The figure shows three views and two pictorial views of one solid part (mm, origin at its lowest corner). Answer the questions. A direction names the side the tool comes from. Coordinates: 2 decimals unless noted, no trailing zeros. Order: outer loops, then holes, each group sorted by start corner. A loop starts at its lowest first (then second) coordinate and runs counter-clockwise, first axis right, second up. Notation, with made-up numbers: (4, 30.25) -> (60, 30.25) arc R23 cw to (60, 44.25) -> close; hole circle Ø9 at (64, -28). An arc over 180 degrees is marked (long way). Return JSON: item names as keys, results as strings.
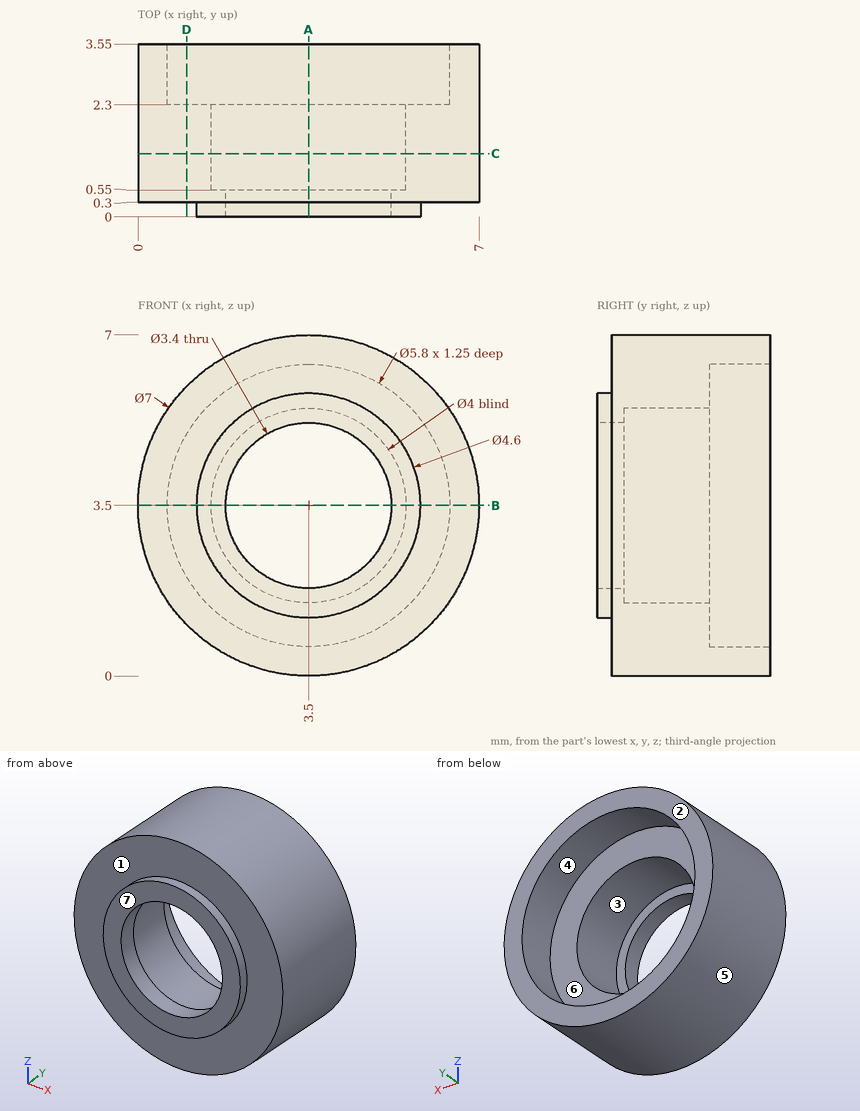
Item 1: The part is cut by section D-D on x = 1. Determine the outline of the cut face in (y, z), plus the area to 3 significant figures.
Answer list:
{"outline": "(0.3, 1.05) -> (3.55, 1.05) -> (3.55, 2.03) -> (2.3, 2.03) -> (2.3, 4.97) -> (3.55, 4.97) -> (3.55, 5.95) -> (0.3, 5.95) -> close", "area": "12.2 mm2"}
Item 2: The part is cut by section C-C on y = 1.3. Determine the outline of the cut face in (x, z), plus the area to 3 significant figures.
Answer list:
{"outline": "circle Ø7 at (3.5, 3.5); hole circle Ø4 at (3.5, 3.5)", "area": "25.9 mm2"}
Item 3: Determine the mould class of the marked faces 4, 5, 6 and 7 for opening direction Z: pulls with the +Z half, pulls with the -Z half, needs draft (parallel to the pull), parting line crosses it, or undercut.
Answer list:
{"face 4": "undercut", "face 5": "parting line crosses it", "face 6": "undercut", "face 7": "needs draft"}
Item 4: The part is cut by section B-B on z = 3.5. Determine the outline of the cut face in (x, y).
Answer list:
{"outline": "(0, 0.3) -> (1.2, 0.3) -> (1.2, 0) -> (1.8, 0) -> (1.8, 0.55) -> (1.5, 0.55) -> (1.5, 2.3) -> (0.6, 2.3) -> (0.6, 3.55) -> (0, 3.55) -> close; (5.2, 0) -> (5.8, 0) -> (5.8, 0.3) -> (7, 0.3) -> (7, 3.55) -> (6.4, 3.55) -> (6.4, 2.3) -> (5.5, 2.3) -> (5.5, 0.55) -> (5.2, 0.55) -> close"}
Item 5: Which of the six approach directions +Z, -Z, +X, -X, +Y, -Y give full straight-line access (tool end or side, diameter ignored) to the marked faces 1, 2 and 3?
Answer list:
{"face 1": "-Y", "face 2": "+Z, -Z, +X, -X, +Y", "face 3": "+Y"}
Item 6: Find the intervals of material crossed by probe 1 along Y at (x, z) = (5.5, 4.5); probe 2 along X at (y, z) = (2.85, 5.5); probe 3 along Y at (x, z) = (4.5, 6.75), in increasing order.
Answer list:
{"probe 1": "0 to 2.3", "probe 2": "0.63 to 1.4, 5.6 to 6.37", "probe 3": "0.3 to 3.55"}
Item 7: The part is cut by section A-A on x = 3.5. Determine the outline of the cut face in (y, z), plus the area to 3 significant figures.
Answer list:
{"outline": "(0, 1.2) -> (0.3, 1.2) -> (0.3, 0) -> (3.55, 0) -> (3.55, 0.6) -> (2.3, 0.6) -> (2.3, 1.5) -> (0.55, 1.5) -> (0.55, 1.8) -> (0, 1.8) -> close; (0, 5.2) -> (0.55, 5.2) -> (0.55, 5.5) -> (2.3, 5.5) -> (2.3, 6.4) -> (3.55, 6.4) -> (3.55, 7) -> (0.3, 7) -> (0.3, 5.8) -> (0, 5.8) -> close", "area": "8.01 mm2"}
Item 8: A flat-ended cylindrical pin translates along its axis: pin 1 (3 mm diameter, centred on x = 3.5, z = 3.5, fed in from +Y). Find the tip coordinate at first contact, or state that the pin passes through.
Answer list:
{"pin 1": "through"}
